Check sheet for the modelled part. Datum: model origin and axes. Units: mm. A direction names the side the tool comes from. Coordinates: 2 decimals unless noted, no trailing zeros. Write each loop counter-clockwise with the first axis right and the second up, starting at its lowest first coordinate (ties: lowest second). Pieces come first, ordered by that corner, then holes. Notation, with made-up numbers: M 44.5,16.5 L 84.5,16.5 A15 cw 84.5,39.5 Z; hole C 32,-21 d6. An arc over 180 degrees is marked long. Answer as CSV lines item,"result". Start each with the question number.
1) Draft check along X on faces 4 (the flat face through (-38, -6, -16)), 5 (the cylindrical face through (4.425, 21.535, 6.386)), 6 (the flat face through (-34, 19, 5)). Enter one of: +X half, -X half, draft (parallel to the pull), parting line (faces both ways), or undercut.
2) Material ranges on L1, parallel to X at y = 22.7, z = 5; L2, parallel to Z at x = -18, y = 21.5; L3, parallel to Y at x = 51, z = 0, recorded low to high. Write a range as [from, to].
3) Section check D-D (x = -2). Record the cut outline in (y, z), and give its area (3 significant figures).
4) Section check A-A (x = -36). State how many separate pieces and enclosed holes the cut face has, and give its area (3 significant figures).
5) Section check C-C (x = -24.5). Record the cut outline in (y, z).
6) Access from +Z, -Z, +X, -X, +Y, -Y to the whole of each face (thin tool, end or side, straight path). Record for faces 1 (the cylindrical face through (51, 0, 5)), 2 (the flat face through (-15, -6.5, -15)), 3 (the cylindrical face through (-39, 21, 2)).
7) Go/stop test with flat-tipped pins: pin 1 Ø0.5 at (y, z) = (3, -14) entering from -X; pin 2 Ø1.5 at (x, y) = (5, -6.5) entering from +Z; pin 3 Ø1 at (x, z) = (-33, -10.5) entering from +Y; pin 4 Ø7 at (y, z) = (0, 0) entering from +X. Record where each tip stops, or that it passes through.
from build123d import *

# Parameters (mm, degrees)
BOSS_EXTRUDE1_REACH = 70.28
SKETCH2_W           = 34
SKETCH2_H           = 10
SKETCH2_W_2         = 30
SKETCH2_H_2         = 6
SKETCH4_W           = 30
SKETCH4_H           = 6
CUT_EXTRUDE4_DEPTH  = 20
SKETCH5_W           = 50
SKETCH5_H           = 10
SKETCH5_R           = 1.5
SKETCH5_W_2         = 30
SKETCH5_H_2         = 6
BOSS_EXTRUDE2_DEPTH = 5
FILLET1_R           = 5
BOSS_EXTRUDE3_REACH = 69.202
SKETCH6_W           = 49
SKETCH6_H           = 1
CHAMFER1_SIZE       = 2


with BuildPart() as part:
    # Sketch1 → Revolve1 (revolve)
    with BuildSketch(Plane.XY, mode=Mode.PRIVATE) as revolve1_sk:
        with BuildLine():
            Line((-41, 13), (24, 15))
            ThreePointArc((24, 15), (26.065530114, 14.762120457), (28, 14))
            Line((28, 14), (46.44629603, 5.214864416))
            ThreePointArc((46.44629603, 5.214864416), (46.719154543, 5.09714106), (47, 5))
            Line((47, 5), (54, 5))
            Line((54, 5), (54, 3))
            Line((54, 3), (52, 3))
            Line((52, 3), (47, 3))
            ThreePointArc((47, 3), (46.274186419, 3.139019493), (45.586334306, 3.409188411))
            Line((45.586334306, 3.409188411), (27.080850933, 12.222512247))
            ThreePointArc((27.080850933, 12.222512247), (25.614773207, 12.813149248), (24.045329018, 13.000448217))
            Line((24.045329018, 13.000448217), (-40.970521752, 10.999960501))
            ThreePointArc((-40.970521752, 10.999960501), (-48.767745467, 7.788589754), (-52, 0))
            Line((-52, 0), (-54, 0))
            ThreePointArc((-54, 0), (-50.192388155, 9.192388155), (-41, 13))
        make_face()
    revolve(revolve1_sk.sketch.rotate(Axis((54, 0, 0), (-1, 0, 0)), 90), axis=Axis((54, 0, 0), (-1, 0, 0)))

    # Boss-Extrude1: up to this cone (the profile starts outside it)
    boss_extrude1_end = Plane(origin=(-15, 0, 0), z_dir=(1, 0, 0)) * Cone(11.197538462, 16.402461538, 169.16, mode=Mode.PRIVATE)
    # Sketch2 → Boss-Extrude1 (add, up to the surface)
    with BuildSketch(Plane(origin=(0, 24, 0), x_dir=(1, 0, 0), z_dir=(0, 1, 0)), mode=Mode.PRIVATE) as boss_extrude1_sk1:
        with Locations((-15, -5)):
            Rectangle(SKETCH2_W, SKETCH2_H)
        with Locations((-15, -5)):
            Rectangle(SKETCH2_W_2, SKETCH2_H_2, mode=Mode.SUBTRACT)
    boss_extrude1_tool1 = extrude(boss_extrude1_sk1.sketch, amount=-BOSS_EXTRUDE1_REACH, mode=Mode.PRIVATE) - boss_extrude1_end
    add(boss_extrude1_tool1.solids().sort_by_distance((-15, 24, 0.354401))[0])

    # Sketch4 → Cut-Extrude4 (cut)
    with BuildSketch(Plane(origin=(0, 24, 0), x_dir=(1, 0, 0), z_dir=(0, 1, 0))):
        with Locations((-15, -5)):
            Rectangle(SKETCH4_W, SKETCH4_H)
    extrude(amount=-CUT_EXTRUDE4_DEPTH, mode=Mode.SUBTRACT)

    # Sketch5 → Boss-Extrude2 (add)
    with BuildSketch(Plane(origin=(0, 24, 0), x_dir=(1, 0, 0), z_dir=(0, 1, 0))):
        with Locations((-15, -5)):
            Rectangle(SKETCH5_W, SKETCH5_H)
        with Locations(Location((-36, -5, 0), (0, 0, 270))):
            Circle(SKETCH5_R, mode=Mode.SUBTRACT)
        with Locations(Location((5, -5, 0), (0, 0, 270))):
            Circle(SKETCH5_R, mode=Mode.SUBTRACT)
        with Locations((-15, -5)):
            Rectangle(SKETCH5_W_2, SKETCH5_H_2, mode=Mode.SUBTRACT)
    extrude(amount=-BOSS_EXTRUDE2_DEPTH)

    # Fillet1
    fillet1_edges = [part.edges().sort_by_distance(p)[0] for p in [
        (10, 21.5, 10),
        (10, 21.5, 0),
        (-40, 21.5, 0),
        (-40, 21.5, 10),
    ]]
    fillet(fillet1_edges, radius=FILLET1_R - 0.0001)  # a hair under: the kernel refuses the full size

    # Boss-Extrude3: up to this cone (the profile starts outside it)
    boss_extrude3_end = Plane(origin=(-14.5, 0, 0), z_dir=(1, 0, 0)) * Cone(11.245618935, 16.385150296, 167.034769231, mode=Mode.PRIVATE)
    # Sketch6 → Boss-Extrude3 (add, up to the surface)
    with BuildSketch(Plane.XY.offset(-17), mode=Mode.PRIVATE) as boss_extrude3_sk1:
        with Locations((-14.5, 6)):
            Rectangle(SKETCH6_W, SKETCH6_H)
    boss_extrude3_tool1 = extrude(boss_extrude3_sk1.sketch, amount=BOSS_EXTRUDE3_REACH, mode=Mode.PRIVATE) - boss_extrude3_end
    add(boss_extrude3_tool1.solids().sort_by_distance((-14.5, 6, -17))[0])
    # Sketch6 → Boss-Extrude3 (add, up to the surface)
    with BuildSketch(Plane.XY.offset(-17), mode=Mode.PRIVATE) as boss_extrude3_sk2:
        with Locations((-14.5, 3)):
            Rectangle(SKETCH6_W, SKETCH6_H)
    boss_extrude3_tool2 = extrude(boss_extrude3_sk2.sketch, amount=BOSS_EXTRUDE3_REACH, mode=Mode.PRIVATE) - boss_extrude3_end
    add(boss_extrude3_tool2.solids().sort_by_distance((-14.5, 3, -17))[0])
    # Sketch6 → Boss-Extrude3 (add, up to the surface)
    with BuildSketch(Plane.XY.offset(-17), mode=Mode.PRIVATE) as boss_extrude3_sk3:
        with Locations((-14.5, 0)):
            Rectangle(SKETCH6_W, SKETCH6_H)
    boss_extrude3_tool3 = extrude(boss_extrude3_sk3.sketch, amount=BOSS_EXTRUDE3_REACH, mode=Mode.PRIVATE) - boss_extrude3_end
    add(boss_extrude3_tool3.solids().sort_by_distance((-14.5, 0, -17))[0])
    # Sketch6 → Boss-Extrude3 (add, up to the surface)
    with BuildSketch(Plane.XY.offset(-17), mode=Mode.PRIVATE) as boss_extrude3_sk4:
        with Locations((-14.5, -3)):
            Rectangle(SKETCH6_W, SKETCH6_H)
    boss_extrude3_tool4 = extrude(boss_extrude3_sk4.sketch, amount=BOSS_EXTRUDE3_REACH, mode=Mode.PRIVATE) - boss_extrude3_end
    add(boss_extrude3_tool4.solids().sort_by_distance((-14.5, -3, -17))[0])
    # Sketch6 → Boss-Extrude3 (add, up to the surface)
    with BuildSketch(Plane.XY.offset(-17), mode=Mode.PRIVATE) as boss_extrude3_sk5:
        with Locations((-14.5, -6)):
            Rectangle(SKETCH6_W, SKETCH6_H)
    boss_extrude3_tool5 = extrude(boss_extrude3_sk5.sketch, amount=BOSS_EXTRUDE3_REACH, mode=Mode.PRIVATE) - boss_extrude3_end
    add(boss_extrude3_tool5.solids().sort_by_distance((-14.5, -6, -17))[0])

    # Chamfer1
    chamfer1_edges = [part.edges().sort_by_distance(p)[0] for p in [
        (10, 6, -17),
        (-39, 6, -17),
        (-39, 3, -17),
        (-39, 0, -17),
        (-39, -3, -17),
        (10, -6, -17),
        (-39, -6, -17),
    ]]
    chamfer(chamfer1_edges, length=CHAMFER1_SIZE)


solid = part.part
Results found:
1,face 4,"-X half"
1,face 5,"undercut"
1,face 6,"draft"
2,L1,"x = [-40, -37.5], [-34.5, -30], [0, 3.5], [6.5, 10]"
2,L2,"z = [0, 2], [8, 10]"
2,L3,"y = [-5, -3], [3, 5]"
3,outline,"M -6.5,-17 L -5.5,-17 L -5.5,-13.09 A14.2 ccw -3.5,-13.76 L -3.5,-17 L -2.5,-17 L -2.5,-13.98 A14.2 ccw -0.5,-14.19 L -0.5,-17 L 0.5,-17 L 0.5,-14.19 A14.2 ccw 2.5,-13.98 L 2.5,-17 L 3.5,-17 L 3.5,-13.76 A14.2 ccw 5.5,-13.09 L 5.5,-17 L 6.5,-17 L 6.5,-12.62 A14.2 ccw 14.2,0 L 24,0 L 24,2 L 12.03,2 A12.2 cw long 9.21,8 L 24,8 L 24,10 L 10.08,10 A14.2 ccw long -6.5,-12.62 Z"
3,area,"216 mm2"
4,separate pieces,"3"
4,enclosed holes,"1"
4,area,"210 mm2"
5,outline,"M -6.5,-17 L -5.5,-17 L -5.5,-12.34 A13.51 ccw -3.5,-13.05 L -3.5,-17 L -2.5,-17 L -2.5,-13.27 A13.51 ccw -0.5,-13.5 L -0.5,-17 L 0.5,-17 L 0.5,-13.5 A13.51 ccw 2.5,-13.27 L 2.5,-17 L 3.5,-17 L 3.5,-13.05 A13.51 ccw 5.5,-12.34 L 5.5,-17 L 6.5,-17 L 6.5,-11.84 A13.51 ccw 13.51,0 L 24,0 L 24,2 L 11.33,2 A11.51 cw long 8.27,8 L 24,8 L 24,10 L 9.08,10 A13.51 ccw long -6.5,-11.84 Z"
6,face 1,"+X"
6,face 2,"-Z, -X, -Y"
6,face 3,"-Z, -X, +Y"
7,pin 1,"stops at x = -39"
7,pin 2,"stops at z = 13.22"
7,pin 3,"stops at y = 8.69"
7,pin 4,"stops at x = 54"
